Build history of the part. All positions in model axes, mm. Give positions to 0.01 mm unless a question says otherwise; leave off trailing zeros. Write each loop counter-clockwise with the first axis right and the second up, starting at its lowest first coordinate (ties: lowest second). Pieces come first, ordered by that corner, then holes.
Autodesk Fusion 360 part; units mm, degrees
sketch "Sketch1" plane through (0, 0, 0) normal (1, 0, 0) x (0, 1, 0)
  circle A0 centre (0, 0) radius 0.5
  line L0 (0.325, -0.325) -> (-0.325, -0.325)
  line L1 (-0.325, -0.325) -> (-0.325, 0.325)
  line L2 (-0.325, 0.325) -> (0.325, 0.325)
  line L3 (0.325, 0.325) -> (0.325, -0.325)
  line L4 (0.325, -0.325) -> (-0.325, 0.325) construction
  line L5 (-0.325, -0.325) -> (0.325, 0.325) construction
  dimension "d1" = 1
  dimension "d2" = 0.65
  dimension "d3" = 0.65
extrude "Extrude1" add sketch "Sketch1" along normal blind 7 contours A0 | L0 L1 L2 L3
sketch "Sketch2" plane through (7, 0, 0) normal (1, 0, 0) x (0, 1, 0)
  circle A0 centre (0, 0) radius 0.5
  line L0 (0.325, -0.325) -> (-0.325, -0.325)
  line L1 (-0.325, -0.325) -> (-0.325, 0.325)
  line L2 (-0.325, 0.325) -> (0.325, 0.325)
  line L3 (0.325, 0.325) -> (0.325, -0.325)
  line L4 (0.325, -0.325) -> (-0.325, 0.325) construction
  line L5 (-0.325, -0.325) -> (0.325, 0.325) construction
  dimension "d8" = 0.65
  dimension "d9" = 0.65
extrude "Extrude2" add sketch "Sketch2" along normal blind 1.905 contours L0 L1 L2 L3
extrude "Extrude3" add sketch "Sketch1" against normal blind 1.905 contours L0 L1 L2 L3
sketch "Sketch3" plane through (0, 0, -0.325) normal (0, 0, -1) x (1, 0, 0)
  line L0 (7, 0.325) -> (7, -0.325)
  line L1 (7, -0.325) -> (8.905, -0.325)
  line L2 (8.905, -0.325) -> (8.905, 0.325)
  line L3 (8.905, 0.325) -> (7, 0.325)
  line L4 (8.905, 0.325) -> (8.255, 0.325)
  line L5 (8.255, 0.325) -> (8.255, -0.325)
  line L6 (8.255, -0.325) -> (8.905, -0.325)
  line L7 (8.905, -0.325) -> (8.905, 0.325)
  line L8 (8.905, 0.325) -> (8.255, -0.325) construction
  line L9 (8.255, 0.325) -> (8.905, -0.325) construction
  point P0 (8.58, 0)
  dimension "d14" = 0.65
  dimension "d15" = 0.65
sketch "Sketch4" plane through (0, 0, -0.325) normal (0, 0, -1) x (1, 0, 0)
  line L0 (0, -0.325) -> (0, 0.325)
  line L1 (0, 0.325) -> (-1.905, 0.325)
  line L2 (-1.905, 0.325) -> (-1.905, -0.325)
  line L3 (-1.905, -0.325) -> (0, -0.325)
  line L4 (-1.255, -0.325) -> (-1.905, -0.325)
  line L5 (-1.905, -0.325) -> (-1.905, 0.325)
  line L6 (-1.905, 0.325) -> (-1.255, 0.325)
  line L7 (-1.255, 0.325) -> (-1.255, -0.325)
  line L8 (-1.255, -0.325) -> (-1.905, 0.325) construction
  line L9 (-1.905, -0.325) -> (-1.255, 0.325) construction
  point P0 (-1.58, 0)
  dimension "d17" = 0.65
  dimension "d18" = 0.65
extrude "Extrude4" add sketch "Sketch4" sketch "Sketch3" along normal blind 7 contours L1 L2 L3 L4 L5 L6 L7 of sketch 2 contours L1 L2 L3 L4 L5 L6 L7
fillet "Fillet1" radius 0.5 2 edges at (-1.255, 0, -0.325) (8.255, 0, -0.325)
fillet "Fillet2" radius 1 2 edges at (-1.905, 0, 0.325) (8.905, 0, 0.325)
fillet "Fillet3" radius 0.2 32 edges at (-1.58, -0.325, -7.325) (-1.255, 0, -7.325) (-1.58, 0.325, -7.325) (-1.905, 0, -7.325) (-1.1086, -0.325, -0.4714) (-1.255, -0.325, -4.075) (-0.3775, -0.325, -0.325) (-0.4525, -0.325, 0.325) (-1.6121, -0.325, 0.0321) (-1.905, -0.325, -4) (-0.4525, 0.325, 0.325) (-1.6121, 0.325, 0.0321) (-1.905, 0.325, -4) (-1.1086, 0.325, -0.4714) (-0.3775, 0.325, -0.325) (-1.255, 0.325, -4.075) (7.4525, -0.325, 0.325) (8.6121, -0.325, 0.0321) (8.905, -0.325, -4) (8.255, -0.325, -4.075) (8.1086, -0.325, -0.4714) (7.3775, -0.325, -0.325) (8.905, 0.325, -4) (8.6121, 0.325, 0.0321) (7.4525, 0.325, 0.325) (8.1086, 0.325, -0.4714) (8.255, 0.325, -4.075) (7.3775, 0.325, -0.325) (8.58, 0.325, -7.325) (8.905, 0, -7.325) (8.58, -0.325, -7.325) (8.255, 0, -7.325)
equation "d1 = jumperWidth"
equation "d2 = d3"
equation "d3 = d1 * 0.65"
equation "jumperWidth = 1 mm"
equation "jumperBaseLenght = 7 mm"
equation "d6 = jumperBaseLenght"
equation "d8 = jumperWidth * 0.65"
equation "d9 = d8"
equation "d14 = jumperWidth * 0.65"
equation "d15 = d14"
equation "d17 = jumperWidth * 0.65"
equation "d18 = d17"
equation "d26 = 0.2 * jumperWidth"
(1) Probe line 1 (X direction, y = 0, z = -5.5) (3 decimals); line 2 (Y direction, x = -0.25, z = 0) (3 decimals); line 3 (Z direction, x = 5.5, y = 0). List the from-to ranges inside material, lowest first.
(2) Saw through at C-C, the plane y = 0. List the corners of the cut face in (x, z) (3 decimals).
(3) Saw through at A-A, the plane z = -5.5. List the corners of the cut face in (x, y) (3 decimals).
(4) Drop flat-ended pins along their axis: pin 1 (1.4 mm diameter, centred on x = 8, z = -2.5, fed in from -Y) (3 decimals); pin 2 (1.5 mm diameter, centred on x = 0.5, z = -1, fed in from +Y); pin 3 (1.9 mm diameter, centred on x = -1, z = -4.5, fed in from +Y) (3 decimals). Give the stop position or say it passes through.
(5) Saw through at D-D, the plane x = 6. List the corners of the cut face in (y, z).
(6) Saw through at B-B, the plane x = -0.5. List the corners of the cut face in (y, z) (3 decimals), plus the area to 3 significant figures.
Computed values:
1. line 1: x = -1.905 to -1.255, 8.255 to 8.905
1. line 2: y = -0.325 to 0.325
1. line 3: z = -0.5 to 0.5
2. outline: (-1.905, -7.125) arc R0.2 ccw to (-1.705, -7.325) - (-1.455, -7.325) arc R0.2 ccw to (-1.255, -7.125) - (-1.255, -0.825) arc R0.5 cw to (-0.755, -0.325) - (0, -0.325) - (0, -0.5) - (7, -0.5) - (7, -0.325) - (7.755, -0.325) arc R0.5 cw to (8.255, -0.825) - (8.255, -7.125) arc R0.2 ccw to (8.455, -7.325) - (8.705, -7.325) arc R0.2 ccw to (8.905, -7.125) - (8.905, -0.675) arc R1 ccw to (7.905, 0.325) - (7, 0.325) - (7, 0.5) - (0, 0.5) - (0, 0.325) - (-0.905, 0.325) arc R1 ccw to (-1.905, -0.675) - close
3. outline: (-1.905, -0.125) arc R0.2 ccw to (-1.705, -0.325) - (-1.455, -0.325) arc R0.2 ccw to (-1.255, -0.125) - (-1.255, 0.125) arc R0.2 ccw to (-1.455, 0.325) - (-1.705, 0.325) arc R0.2 ccw to (-1.905, 0.125) - close; (8.255, -0.125) arc R0.2 ccw to (8.455, -0.325) - (8.705, -0.325) arc R0.2 ccw to (8.905, -0.125) - (8.905, 0.125) arc R0.2 ccw to (8.705, 0.325) - (8.455, 0.325) arc R0.2 ccw to (8.255, 0.125) - close
4. pin 1: stops at y = -0.325
4. pin 2: stops at y = 0.43
4. pin 3: stops at y = 0.325
5. outline: circle Ø1 at (0, 0)
6. outline: (-0.325, -0.125) arc R0.2 ccw to (-0.125, -0.325) - (0.125, -0.325) arc R0.2 ccw to (0.325, -0.125) - (0.325, 0.125) arc R0.2 ccw to (0.125, 0.325) - (-0.125, 0.325) arc R0.2 ccw to (-0.325, 0.125) - close
6. area: 0.388 mm2
